For this review, take the finished solid that the model builds, in its own axes (mm). Face numbers are marked on the shaded views. A direction names the side the tool comes from. Give positions to 0.01 mm unless a question says otherwise; leave off trailing zeros. Order: outer loops, then holes, each group sorted by start corner. A loop starts at its lowest first (then second) coordinate and runs counter-clockwise, first axis right, second up. Notation, with made-up numbers: (53.25, -19) - (104.25, -19) arc R22 cw to (104.25, 13) - close; hole circle Ø7 at (25.25, 15.5). An arc over 180 degrees is marked (long way). Use a Markdown table: item, result. Add a question column.
1) Wall thickness on L1, parallel to Y at x = 168.5, z = 265; L2, parallel to X at y = 50, z = 30; L3, parallel to Z at x = -10, y = 44 (3 decimals): over which ranges is each line inside the solid? List them lowest first.
2) We need section A-A on z = 220. Write out the cut boundary in (x, y).
3) We need section D-D on y = 54.5. Write out the cut boundary in (x, z), then the cut area to 3 significant figures.
4) We need section B-B on y = 22.5. Write out the cut boundary in (x, z).
5) Mouldability with a two-part tool opening along X and no side actions: class the marked faces 4, 5 and 6 as released by +X, released by -X, zero draft, split by the parting line, or undercut.
6) Clearance check with flat-ended pins moving along their axes: P1, Ø12, axis at x = -10.5, z = 96, coming from the +Y side; P2, Ø5.5, axis at x = 160, z = 170, coming from the -Y side; P3, Ø8, axis at x = 49, z = 64, coming from the +Y side. State where each tip first meets the part, or that it passes through.
7) We need section C-C on z = 19.5. Write out the cut boundary in (x, y), then the cut area to 3 significant figures.
8) Machinability: for the marked faces 1, 2 and 3, which of the approach directions +Z, -Z, +X, -X, +Y, -Y give a long, thin tool a straight path to every point of the face, cutting with its end or side? Answer none if there is none.
```python
from build123d import *

# Parameters (mm, degrees)
SKETCH1_W           = 10
SKETCH1_H           = 5
BOSS_EXTRUDE1_DEPTH = 200
SKETCH2_R           = 2.38125
CUT_EXTRUDE1_DEPTH  = 200
SKETCH3_W           = 10
SKETCH3_H           = 30
SKETCH3_H_2         = 5
BOSS_EXTRUDE2_DEPTH = 100
CUT_EXTRUDE2_DEPTH  = 100
BOSS_EXTRUDE5_START = -15
SKETCH5_R           = 6.35
BOSS_EXTRUDE5_DEPTH = 15
SKETCH6_R           = 6.35
BOSS_EXTRUDE6_DEPTH = 5
BOSS_EXTRUDE7_START = -200
BOSS_EXTRUDE7_DEPTH = 200
SKETCH8_R           = 6.35
BOSS_EXTRUDE8_DEPTH = 9
SKETCH9_R           = 6.35
BOSS_EXTRUDE9_DEPTH = 9
SKETCH10_R          = 6.35
CUT_EXTRUDE3_DEPTH  = 5
SKETCH11_R          = 6.35
CUT_EXTRUDE4_DEPTH  = 5
SKETCH12_R          = 2.38125
CUT_EXTRUDE5_DEPTH  = 66


with BuildPart() as part:
    # Sketch1 → Boss-Extrude1 (new body)
    with BuildSketch(Plane.XY):
        with Locations((-10, 62.5)):
            Rectangle(SKETCH1_W, SKETCH1_H)
        with BuildLine():
            Line((90, 0), (60, 0))
            ThreePointArc((60, 0), (17.573593, 17.573593), (0, 60))
            Line((0, 60), (0, 65))
            Line((0, 65), (-5, 65))
            Line((-5, 65), (-5, 60))
            ThreePointArc((-5, 60), (14.038059, 14.038059), (60, -5))
            Line((60, -5), (90, -5))
            ThreePointArc((90, -5), (135.961941, 14.038059), (155, 60))
            Line((155, 60), (155, 65))
            Line((155, 65), (150, 65))
            Line((150, 65), (150, 60))
            ThreePointArc((150, 60), (132.426407, 17.573593), (90, 0))
        make_face()
        with Locations((160, 62.5)):
            Rectangle(SKETCH1_W, SKETCH1_H)
    extrude(amount=BOSS_EXTRUDE1_DEPTH)

    # Sketch2 → Cut-Extrude1 (cut)
    with BuildSketch(Plane(origin=(0, 65, 0), x_dir=(1, 0, 0), z_dir=(0, 1, 0))):
        with Locations((-10, -170)):
            Circle(SKETCH2_R)
        with Locations((-10, -30)):
            Circle(SKETCH2_R)
        with Locations((160, -30)):
            Circle(SKETCH2_R)
        with Locations((160, -170)):
            Circle(SKETCH2_R)
    extrude(amount=-CUT_EXTRUDE1_DEPTH, mode=Mode.SUBTRACT)

    # Sketch3 → Boss-Extrude2 (add)
    with BuildSketch(Plane.XY.offset(200)):
        with Locations((-10, 45)):
            Rectangle(SKETCH3_W, SKETCH3_H)
        with Locations((-10, 62.5)):
            Rectangle(SKETCH3_W, SKETCH3_H_2)
        with Locations((-10, 67.5)):
            Rectangle(SKETCH3_W, SKETCH3_H_2)
        with Locations((-10, 85)):
            Rectangle(SKETCH3_W, SKETCH3_H)
    extrude(amount=BOSS_EXTRUDE2_DEPTH)

    # Sketch4 → Cut-Extrude2 (cut)
    with BuildSketch(Plane(origin=(-5, 0, 0), x_dir=(0, 0, -1), z_dir=(1, 0, 0))):
        with BuildLine():
            ThreePointArc((-260.509872, 69.490128), (-269.490128, 69.490128), (-269.490128, 60.509872))
            Line((-269.490128, 60.509872), (-260.509872, 69.490128))
        make_face()
        with BuildLine():
            Line((-260.509872, 69.490128), (-269.490128, 60.509872))
            ThreePointArc((-269.490128, 60.509872), (-262.56996, 59.133365), (-258.65, 65))
            ThreePointArc((-258.65, 65), (-259.133365, 67.43004), (-260.509872, 69.490128))
        make_face()
        with BuildLine():
            Line((-300, 30), (-265.01, 30))
            ThreePointArc((-265.01, 30), (-278.400093, 32.663455), (-289.751666, 40.248334))
            Line((-289.751666, 40.248334), (-300, 30))
        make_face()
        with BuildLine():
            Line((-300, 30), (-289.751666, 40.248334))
            ThreePointArc((-289.751666, 40.248334), (-297.336545, 51.599907), (-300, 64.99))
            Line((-300, 64.99), (-300, 30))
        make_face()
        with BuildLine():
            ThreePointArc((-300, 65.01), (-289.751666, 89.751666), (-265.01, 100))
            Line((-265.01, 100), (-300, 100))
            Line((-300, 100), (-300, 65.01))
        make_face()
    extrude(amount=-CUT_EXTRUDE2_DEPTH, mode=Mode.SUBTRACT)

    # Sketch5 → Boss-Extrude5 (add)
    with BuildSketch(Plane(origin=(165, 0, 0), x_dir=(0, 0, -1), z_dir=(1, 0, 0)).offset(BOSS_EXTRUDE5_START)):
        with BuildLine():
            Line((-300, 65.01), (-300, 64.99))
            ThreePointArc((-300, 64.99), (-289.751666, 40.248334), (-265.01, 30))
            Line((-265.01, 30), (-200, 30))
            Line((-200, 30), (-200, 60))
            Line((-200, 60), (-200, 65))
            Line((-200, 65), (-200, 100))
            Line((-200, 100), (-265.01, 100))
            ThreePointArc((-265.01, 100), (-289.751666, 89.751666), (-300, 65.01))
        make_face()
        with Locations((-265, 65)):
            Circle(SKETCH5_R, mode=Mode.SUBTRACT)
    extrude(amount=BOSS_EXTRUDE5_DEPTH)

    # Sketch6 → Boss-Extrude6 (add)
    with BuildSketch(Plane(origin=(-5, 0, 0), x_dir=(0, 0, -1), z_dir=(1, 0, 0))):
        with BuildLine():
            Line((-300, 65.01), (-300, 64.99))
            ThreePointArc((-300, 64.99), (-289.751666, 40.248334), (-265.01, 30))
            Line((-265.01, 30), (-200, 30))
            Line((-200, 30), (-200, 60))
            Line((-200, 60), (-200, 65))
            Line((-200, 65), (-200, 100))
            Line((-200, 100), (-265.01, 100))
            ThreePointArc((-265.01, 100), (-289.751666, 89.751666), (-300, 65.01))
        make_face()
        with Locations((-265, 65)):
            Circle(SKETCH6_R, mode=Mode.SUBTRACT)
    extrude(amount=BOSS_EXTRUDE6_DEPTH)

    # Sketch7 → Boss-Extrude7 (add)
    with BuildSketch(Plane(origin=(0, 0, 0), x_dir=(-1, 0, 0), z_dir=(0, 0, -1)).offset(BOSS_EXTRUDE7_START)):
        with BuildLine():
            Line((-150, 35), (-150, 30))
            Line((-150, 30), (-147.662813, 30))
            ThreePointArc((-147.662813, 30), (-148.8845, 32.475182), (-150, 35))
        make_face()
        with BuildLine():
            Line((-165, 60), (-165, 30))
            Line((-165, 30), (-150, 30))
            Line((-150, 30), (-150, 35))
            ThreePointArc((-150, 35), (-153.737744, 47.252451), (-155, 60))
            Line((-155, 60), (-165, 60))
        make_face()
        with BuildLine():
            ThreePointArc((0, 35), (-1.1155, 32.475182), (-2.337187, 30))
            Line((-2.337187, 30), (0, 30))
            Line((0, 30), (0, 35))
        make_face()
        with BuildLine():
            Line((0, 35), (0, 30))
            Line((0, 30), (5, 30))
            Line((5, 30), (15, 30))
            Line((15, 30), (15, 60))
            Line((15, 60), (5, 60))
            ThreePointArc((5, 60), (3.737744, 47.252451), (0, 35))
        make_face()
    extrude(amount=BOSS_EXTRUDE7_DEPTH)

    # Sketch8 → Boss-Extrude8 (add)
    with BuildSketch(Plane(origin=(165, 0, 0), x_dir=(0, 0, -1), z_dir=(1, 0, 0))):
        with BuildLine():
            Line((-200, 65), (-200, 100))
            Line((-200, 100), (-265.01, 100))
            ThreePointArc((-265.01, 100), (-289.751666, 89.751666), (-300, 65.01))
            Line((-300, 65.01), (-300, 64.99))
            ThreePointArc((-300, 64.99), (-289.751666, 40.248334), (-265.01, 30))
            Line((-265.01, 30), (-200, 30))
            Line((-200, 30), (-200, 65))
        make_face()
        with Locations((-265, 65)):
            Circle(SKETCH8_R, mode=Mode.SUBTRACT)
    extrude(amount=BOSS_EXTRUDE8_DEPTH)

    # Sketch9 → Boss-Extrude9 (add)
    with BuildSketch(Plane.ZY.offset(15)):
        with BuildLine():
            Line((265.01, 100), (200, 100))
            Line((200, 100), (200, 65))
            Line((200, 65), (200, 30))
            Line((200, 30), (265.01, 30))
            ThreePointArc((265.01, 30), (289.751666, 40.248334), (300, 64.99))
            Line((300, 64.99), (300, 65.01))
            ThreePointArc((300, 65.01), (289.751666, 89.751666), (265.01, 100))
        make_face()
        with Locations((265, 65)):
            Circle(SKETCH9_R, mode=Mode.SUBTRACT)
    extrude(amount=BOSS_EXTRUDE9_DEPTH)

    # Sketch10 → Cut-Extrude3 (cut)
    with BuildSketch(Plane.ZY.offset(-150)):
        with BuildLine():
            Line((200, 60), (200, 65))
            Line((200, 65), (200, 100))
            Line((200, 100), (265.01, 100))
            ThreePointArc((265.01, 100), (289.751666, 89.751666), (300, 65.01))
            Line((300, 65.01), (300, 64.99))
            ThreePointArc((300, 64.99), (289.751666, 40.248334), (265.01, 30))
            Line((265.01, 30), (200, 30))
            Line((200, 30), (200, 60))
        make_face()
        with Locations((265, 65)):
            Circle(SKETCH10_R, mode=Mode.SUBTRACT)
    extrude(amount=-CUT_EXTRUDE3_DEPTH, mode=Mode.SUBTRACT)

    # Sketch11 → Cut-Extrude4 (cut)
    with BuildSketch(Plane(origin=(0, 0, 0), x_dir=(0, 0, -1), z_dir=(1, 0, 0))):
        with BuildLine():
            Line((-200, 60), (-200, 65))
            Line((-200, 65), (-200, 100))
            Line((-200, 100), (-265.01, 100))
            ThreePointArc((-265.01, 100), (-289.751666, 89.751666), (-300, 65.01))
            Line((-300, 65.01), (-300, 64.99))
            ThreePointArc((-300, 64.99), (-289.751666, 40.248334), (-265.01, 30))
            Line((-265.01, 30), (-200, 30))
            Line((-200, 30), (-200, 60))
        make_face()
        with Locations((-265, 65)):
            Circle(SKETCH11_R, mode=Mode.SUBTRACT)
    extrude(amount=-CUT_EXTRUDE4_DEPTH, mode=Mode.SUBTRACT)

    # Sketch12 → Cut-Extrude5 (cut, through all)
    with BuildSketch(Plane(origin=(0, 60, 0), x_dir=(1, 0, 0), z_dir=(0, 1, 0))):
        with Locations((160, -30)):
            Circle(SKETCH12_R)
        with Locations((-10, -170)):
            Circle(SKETCH12_R)
        with Locations((-10, -30)):
            Circle(SKETCH12_R)
        with Locations((160, -170)):
            Circle(SKETCH12_R)
    extrude(amount=-CUT_EXTRUDE5_DEPTH, mode=Mode.SUBTRACT)


solid = part.part
```
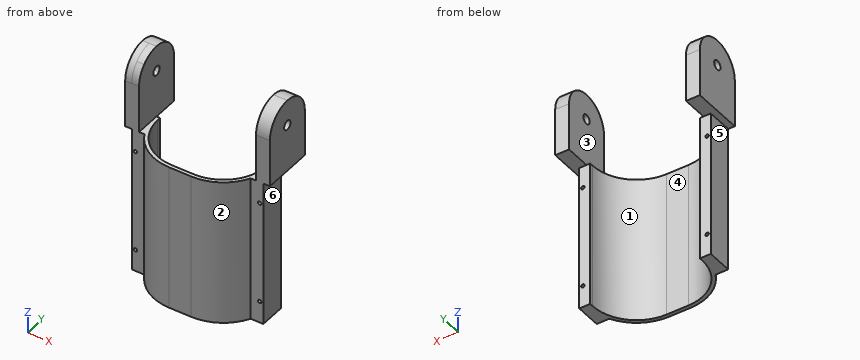
Checked values:
| question | item | result |
|---|---|---|
| 1 | L1 | 30 to 58.65, 71.35 to 100 |
| 1 | L2 | -15 to -12.38, -7.62 to 0.84, 149.16 to 157.62, 162.38 to 165 |
| 1 | L3 | 0 to 27.619, 32.381 to 167.619, 172.381 to 293.005 |
| 2 | outline | (-24, 30) - (-5, 30) - (-5, 100) - (-24, 100) - close; (155, 30) - (174, 30) - (174, 100) - (155, 100) - close |
| 3 | outline | (-24, 200) - (-15, 200) - (-15, 0) - (0.25, 0) - (0.25, 200) - (-5, 200) - (-5, 298.39) - (-24, 298.39) - close; (149.75, 0) - (165, 0) - (165, 200) - (174, 200) - (174, 298.39) - (155, 298.39) - (155, 200) - (149.75, 200) - close; hole circle Ø4.76 at (-10, 30); hole circle Ø4.76 at (-10, 170); hole circle Ø4.76 at (160, 30); hole circle Ø4.76 at (160, 170) |
| 3 | area | 9,770 mm² |
| 4 | outline | (6.91, 0) - (13.16, 0) - (13.16, 200) - (6.91, 200) - close; (136.84, 0) - (143.09, 0) - (143.09, 200) - (136.84, 200) - close |
| 5 | face 4 | undercut |
| 5 | face 5 | released by -X |
| 5 | face 6 | released by +X |
| 6 | P1 | y = 65 |
| 6 | P2 | y = 30 |
| 6 | P3 | y = 1.91 |
| 7 | outline | (-15, 30) - (2.34, 30) arc R65 ccw to (60, -5) - (90, -5) arc R65 ccw to (147.66, 30) - (165, 30) - (165, 65) - (150, 65) - (150, 60) arc R60 cw to (90, 0) - (60, 0) arc R60 cw to (0, 60) - (0, 65) - (-15, 65) - close |
| 7 | area | 2,030 mm² |
| 8 | face 1 | +Z, -Z, +Y |
| 8 | face 2 | +Z, -Z, +X, -Y |
| 8 | face 3 | +Z, +Y, -Y |
